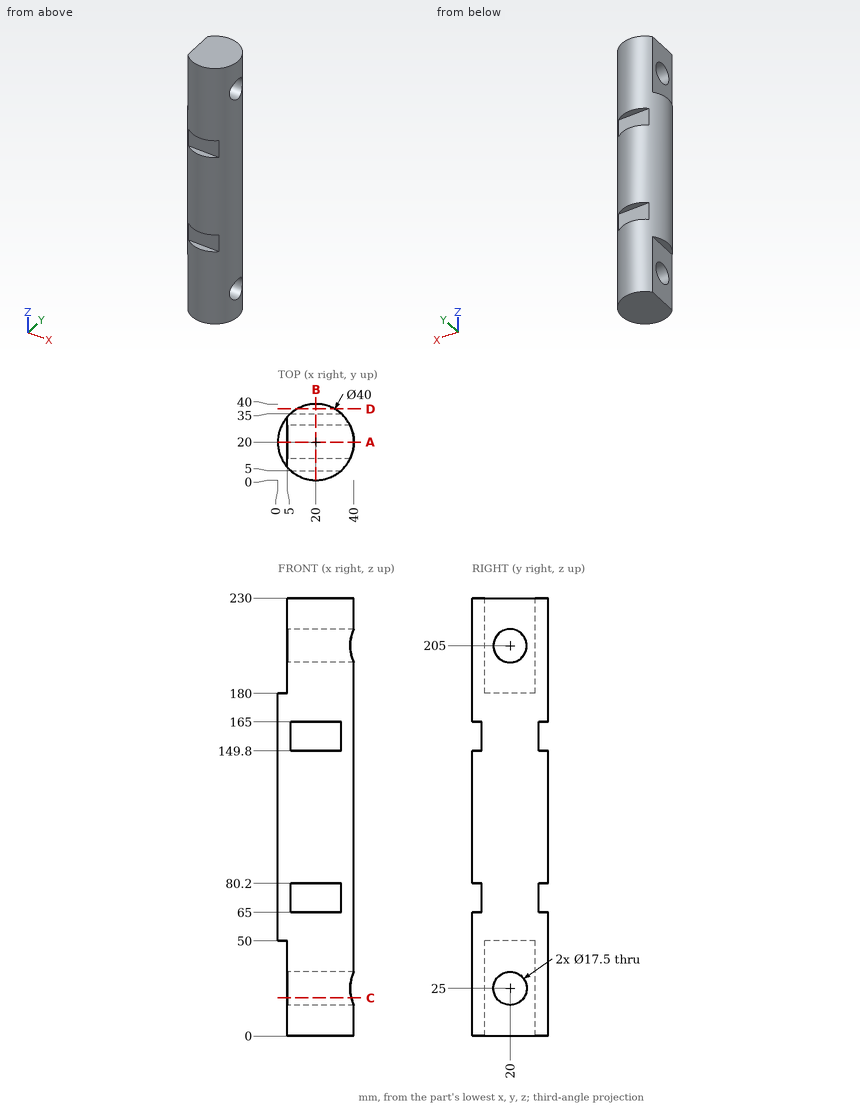
Input: dimensioned drawing with shaded views. Units: mm. Origin: part minimum x, y, z. Coordinates: 2 decimals unless noted, no trailing zeros. Order: outer loops, then holes, each group sorted by start corner. A loop starts at its lowest first (then second) coordinate and runs counter-clockwise, first axis right, second up. Notation, with made-up numbers: (18, 34) - (58, 34) arc R18 ccw to (58, 42) - close; hole circle Ø5 at (24.25, 18.25). An arc over 180 degrees is marked (long way). Put each result on its own line as item: value.
1. Cut plane D-D on y = 37.5. Return the cut outline in (x, z), then the cut area to 3 significant figures.
Report:
outline: (10.32, 0) - (29.68, 0) - (29.68, 65) - (10.32, 65) - close; (10.32, 80.2) - (29.68, 80.2) - (29.68, 149.8) - (10.32, 149.8) - close; (10.32, 165) - (29.68, 165) - (29.68, 230) - (10.32, 230) - close
area: 3,870 mm2
2. Contact query for flat-ended pins moving along their axis: pin 1 Ø2.5 at (x, y) = (3.5, 26) entering from +Z; pin 2 Ø7.5 at (x, z) = (21.5, 153.5) entering from -Y; pin 3 Ø16.5 at (x, z) = (21.5, 74) entering from +Y. Output: stop coordinate, or through.
Report:
pin 1: stops at z = 180
pin 2: stops at y = 0.02
pin 3: stops at y = 40
3. Cut plane B-B on x = 20. Return the cut outline in (y, z).
Report:
outline: (0, 0) - (40, 0) - (40, 65) - (35, 65) - (35, 80.2) - (40, 80.2) - (40, 149.8) - (35, 149.8) - (35, 165) - (40, 165) - (40, 230) - (0, 230) - (0, 165) - (5, 165) - (5, 149.8) - (0, 149.8) - (0, 80.2) - (5, 80.2) - (5, 65) - (0, 65) - close; hole circle Ø17.5 at (20, 25); hole circle Ø17.5 at (20, 205)
4. Line query: line 1 along Z through (x, y) = (32, 19); line 2 along Y through (x, z) = (19, 205); line 3 along Z through (x, y) = (3.5, 14). Output: solid intervals per line, ascending.
Report:
line 1: z = 0 to 16.31, 33.69 to 196.31, 213.69 to 230
line 2: y = 0.03 to 11.25, 28.75 to 39.97
line 3: z = 50 to 180
5. Cut plane C-C on z = 20. Return the cut outline in (x, y), then the cut area to 3 significant figures.
Report:
outline: (5, 6.77) arc R20 ccw to (38.67, 12.82) - (5, 12.82) - close; (5, 27.18) - (38.67, 27.18) arc R20 ccw to (5, 33.23) - close
area: 670 mm2
6. Cut plane A-A on y = 20. Return the cut outline in (x, z), then the cut area to 4 significant figures.
Report:
outline: (0, 50) - (5, 50) - (5, 33.75) - (40, 33.75) - (40, 196.25) - (5, 196.25) - (5, 180) - (0, 180) - close; (5, 0) - (40, 0) - (40, 16.25) - (5, 16.25) - close; (5, 213.75) - (40, 213.75) - (40, 230) - (5, 230) - close
area: 7,475 mm2
